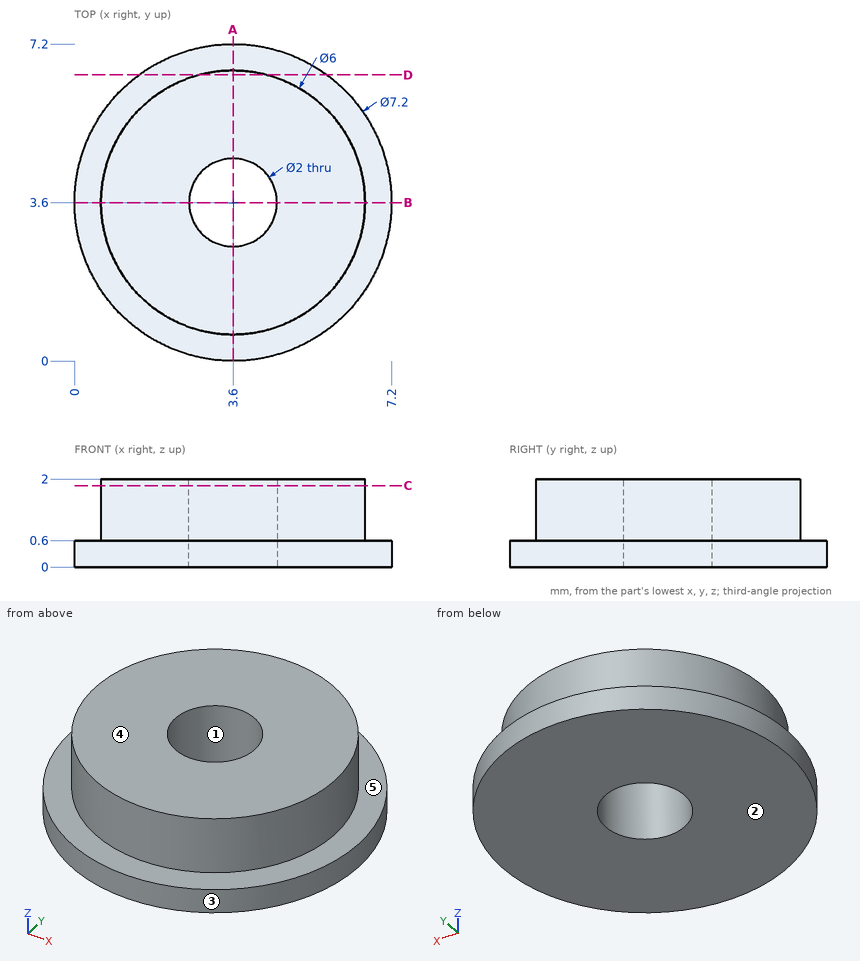
Design review of the part shown in the three views and the two pictorial views. Dimensions are in mm from the part's minimum x, y and z. A direction names the side the tool comes from. Round coordinates to 2 decimals unless told otherwise and drop trailing zeros. Loops run counter-clockwise (first coordinate to the right, second up) from the corner with the lowest first, then second, coordinate; pieces in that order, holes last. Notation, with made-up numbers: (1.25, 31.5) -> (26.25, 31.5) arc R26 cw to (26.25, 64.5) -> close; hole circle Ø1 at (66, 87). An arc over 180 degrees is marked (long way). Return JSON: item names as keys, results as strings.
(1) For the marked faces 4 and 5, list the 3-axis set-ups (+Z, -Z, +X, -X, +Y, -Y) from which the entire face can be reached by the end or side of a thin tool; tool diameter is ignored.
Solved:
{"face 4": "+Z, +X, -X, +Y, -Y", "face 5": "+Z"}
(2) Add section A-A on x = 3.6. Write out the cut boundary in (y, z).
Solved:
{"outline": "(0, 0) -> (2.6, 0) -> (2.6, 2) -> (0.6, 2) -> (0.6, 0.6) -> (0, 0.6) -> close; (4.6, 0) -> (7.2, 0) -> (7.2, 0.6) -> (6.6, 0.6) -> (6.6, 2) -> (4.6, 2) -> close"}
(3) The part is to be moulded in two halves that separate along Y. For the marked faces 1, 2 and 3, say which applies: released by +Y, released by -Y, zero draft, split by the parting line, or undercut.
Solved:
{"face 1": "undercut", "face 2": "zero draft", "face 3": "split by the parting line"}
(4) Add section C-C on z = 1.85. Write out the cut boundary in (x, y), plus the area to 3 significant figures.
Solved:
{"outline": "circle Ø6 at (3.6, 3.6); hole circle Ø2 at (3.6, 3.6)", "area": "25.1 mm2"}
(5) For line 1 (Y direction, x = 3.6, z = 0.9); line 2 (Z direction, x = 4.75, y = 6.5); line 3 (X direction, y = 3.25, z = 1.2), list the stretches that pass through material, from the lowest coordinate up.
Solved:
{"line 1": "0.6 to 2.6, 4.6 to 6.6", "line 2": "0 to 0.6", "line 3": "0.62 to 2.66, 4.54 to 6.58"}
(6) For pin 1 (1 mm diameter, centred on y = 1, z = 1.5, fed in from -X), flat-tipped, find the tip position at first contact; note if it passes through.
Solved:
{"pin 1": "x = 1.46"}
(7) Add section D-D on y = 6.5. Write out the cut boundary in (x, z).
Solved:
{"outline": "(1.47, 0) -> (5.73, 0) -> (5.73, 0.6) -> (4.37, 0.6) -> (4.37, 2) -> (2.83, 2) -> (2.83, 0.6) -> (1.47, 0.6) -> close"}
